```python
from build123d import *

# Parameters (mm, degrees)
F1_DEPTH = 580
F3_W     = 160
F3_H     = 100
F3_R     = 6
F4_DEPTH = 10
F6_W     = 160
F6_H     = 100
F6_R     = 6
F7_DEPTH = 10


with BuildPart() as f1:
    # F0 (on Front) → F1 (new body)
    with BuildSketch(Plane.XZ):
        with BuildLine():
            ThreePointArc((50, 45), (48.5355339059, 48.5355339059), (45, 50))
            Line((45, 50), (-45, 50))
            ThreePointArc((-45, 50), (-48.5355339059, 48.5355339059), (-50, 45))
            Line((-50, 45), (-50, -45))
            ThreePointArc((-50, -45), (-48.5355339059, -48.5355339059), (-45, -50))
            Line((-45, -50), (45, -50))
            ThreePointArc((45, -50), (48.5355339059, -48.5355339059), (50, -45))
            Line((50, -45), (50, 45))
        make_face()
        with BuildLine():
            ThreePointArc((-47, 45), (-46.4142135624, 46.4142135624), (-45, 47))
            Line((-45, 47), (45, 47))
            ThreePointArc((45, 47), (46.4142135624, 46.4142135624), (47, 45))
            Line((47, 45), (47, -45))
            ThreePointArc((47, -45), (46.4142135624, -46.4142135624), (45, -47))
            Line((45, -47), (-45, -47))
            ThreePointArc((-45, -47), (-46.4142135624, -46.4142135624), (-47, -45))
            Line((-47, -45), (-47, 45))
        make_face(mode=Mode.SUBTRACT)
    extrude(amount=-F1_DEPTH)

    # F3 (on offset) → F4 (join)
    with BuildSketch(Plane.XZ.offset(10)):
        Rectangle(F3_W, F3_H)
        with Locations((-64, -34)):
            Circle(F3_R, mode=Mode.SUBTRACT)
        with Locations((64, -34)):
            Circle(F3_R, mode=Mode.SUBTRACT)
        with Locations((-64, 34)):
            Circle(F3_R, mode=Mode.SUBTRACT)
        with Locations((64, 34)):
            Circle(F3_R, mode=Mode.SUBTRACT)
    extrude(amount=-F4_DEPTH)

    # F6 (on offset) → F7 (join)
    with BuildSketch(Plane(origin=(0, 590, 0), x_dir=(-1, 0, 0), z_dir=(0, 1, 0))):
        Rectangle(F6_W, F6_H)
        with Locations((-64, -34)):
            Circle(F6_R, mode=Mode.SUBTRACT)
        with Locations((64, -34)):
            Circle(F6_R, mode=Mode.SUBTRACT)
        with Locations((-64, 34)):
            Circle(F6_R, mode=Mode.SUBTRACT)
        with Locations((64, 34)):
            Circle(F6_R, mode=Mode.SUBTRACT)
    extrude(amount=-F7_DEPTH)


solid = f1.part
```
Input: part model. Units: mm. Frame: model coordinates. A direction names the side the tool comes from. Round coordinates to 2 decimals unless told otherwise and drop trailing zeros. Write each loop counter-clockwise with the first axis right and the second up, starting at its lowest first coordinate (ties: lowest second). Pieces come first, ordered by that corner, then holes. Notation, with made-up numbers: (56.5, -14.5) - (61.5, -14.5) arc R28 cw to (61.5, 24.5) - close; hole circle Ø3 at (30.5, 84.25). An arc over 180 degrees is marked (long way). Write item = value, one per line.
(1) Material intervals for probe 1 along Z at (x, y) = (64, -4.5); probe 2 along Y at (x, z) = (-0.5, 4); probe 3 along X at (y, z) = (133, -22), sorted ascending.
Geometry check:
probe_1 = -50 to -40, -28 to 28, 40 to 50
probe_2 = -10 to 0, 580 to 590
probe_3 = -50 to -47, 47 to 50
(2) Section query C-C on y = 102.5. Output: boundary loops of the cut face in (x, z), then the cut area to 3 significant figures.
Geometry check:
outline = (-50, -45) arc R5 ccw to (-45, -50) - (45, -50) arc R5 ccw to (50, -45) - (50, 45) arc R5 ccw to (45, 50) - (-45, 50) arc R5 ccw to (-50, 45) - close; hole (-47, -45) arc R2 ccw to (-45, -47) - (45, -47) arc R2 ccw to (47, -45) - (47, 45) arc R2 ccw to (45, 47) - (-45, 47) arc R2 ccw to (-47, 45) - close
area = 1,150 mm^2
(3) Contact query for flat-ended pins moving along their axis: pin 1 Ø9.5 at (x, z) = (-64, 34) entering from +Y; pin 2 Ø6 at (y, z) = (167.5, 29.5) entering from +X; pin 3 Ø8 at (y, z) = (51, 6) entering from -X. Output: stop coordinate, or through.
Geometry check:
pin_1 = through
pin_2 = 50
pin_3 = -50
(4) Pull-direction query (Z, two-part tool) for faces 4 (the flat face through (1, 294, -50)), 5 (the flat face through (-66, 580, 1)), 6 (the flat face through (-1, 0, 1)); classes: +Z half, -Z half, draft (parallel to the pull), parting line (faces both ways), or undercut.
Geometry check:
face_4 = -Z half
face_5 = draft
face_6 = undercut
(5) Section query A-A on z = 34. State how many separate pieces and enclosed holes the cut face has, then the cut area to 3 significant figures.
Geometry check:
separate_pieces = 5
enclosed_holes = 1
area = 6,200 mm^2
(6) Section query D-D on x = -64. Output: boundary loops of the cut face in (y, z).
Geometry check:
outline = (-10, -50) - (0, -50) - (0, -40) - (-10, -40) - close; (-10, -28) - (0, -28) - (0, 28) - (-10, 28) - close; (-10, 40) - (0, 40) - (0, 50) - (-10, 50) - close; (580, -50) - (590, -50) - (590, -40) - (580, -40) - close; (580, -28) - (590, -28) - (590, 28) - (580, 28) - close; (580, 40) - (590, 40) - (590, 50) - (580, 50) - close
(7) Section query B-B on x = 17.5. Output: boundary loops of the cut face in (y, z).
Geometry check:
outline = (-10, -50) - (590, -50) - (590, 50) - (-10, 50) - close; hole (0, -47) - (580, -47) - (580, 47) - (0, 47) - close
(8) Access query for faces 1 (the flat face through (50, 286, -1)), 2 (the flat face through (1, 294, 50)), 3 (the flat face through (-1, 286, 47)). Directions: +Z, -Z, +X, -X, +Y, -Y. A direction counts if a zero-diameter tool reaches every point of the face in a straight line with its end or side. Return the directions, or none.
Geometry check:
face_1 = +Z, -Z, +X
face_2 = +Z, +X, -X, +Y, -Y
face_3 = none
